Read the model definition and answer for the solid it produces. Units are mm, in the model's axes. A direction names the side the tool comes from. Coordinates: 2 decimals unless noted, no trailing zeros. Order: outer loops, then holes, each group sorted by start corner. A loop starts at its lowest first (then second) coordinate and runs counter-clockwise, first axis right, second up. Notation, with made-up numbers: (-23.5, 1.5) -> (5.5, 1.5) arc R29 ccw to (5.5, 31.5) -> close; hole circle Ø3 at (-18.75, 11). An arc over 180 degrees is marked (long way). Answer in a Markdown table with one row per item.
from build123d import *

# Parameters (mm, degrees)
SKETCH1_W           = 50
SKETCH1_H           = 25
BOSS_EXTRUDE1_DEPTH = 3
BOSS_EXTRUDE2_DEPTH = 42
SKETCH3_R           = 1.7
CUT_EXTRUDE1_DEPTH  = 71.774289117
FILLET2_R           = 4
FILLET3_R           = 4


with BuildPart() as part:
    # Sketch1 → Boss-Extrude1 (new body)
    with BuildSketch(Plane.XY):
        with Locations((25, -12.5)):
            Rectangle(SKETCH1_W, SKETCH1_H)
    extrude(amount=-BOSS_EXTRUDE1_DEPTH)

    # Sketch2 → Boss-Extrude2 (add)
    with BuildSketch(Plane(origin=(0, 0, -3), x_dir=(-1, 0, 0), z_dir=(0, 0, -1))):
        Polygon((-25, -25), (-29, -25), (-29, -22), (-25, -22), (-21, -22), (-21, -25), align=None)
    extrude(amount=BOSS_EXTRUDE2_DEPTH)

    # Sketch3 → Cut-Extrude1 (cut, through all)
    with BuildSketch(Plane(origin=(0, -22, 0), x_dir=(1, 0, 0), z_dir=(0, 1, 0))):
        with Locations(Location((25, 42, 0), (0, 0, 270))):
            Circle(SKETCH3_R)
        with Locations(Location((25, 15.3, 0), (0, 0, 270))):
            Circle(SKETCH3_R)
    extrude(amount=-CUT_EXTRUDE1_DEPTH, mode=Mode.SUBTRACT)

    # Fillet2
    fillet2_edges = [part.edges().sort_by_distance(p)[0] for p in [
        (29, -23.5, -45),
    ]]
    fillet(fillet2_edges, radius=FILLET2_R)

    # Fillet3
    fillet3_edges = [part.edges().sort_by_distance(p)[0] for p in [
        (21, -23.5, -45),
    ]]
    fillet(fillet3_edges, radius=FILLET3_R - 0.0001)  # a hair under: the kernel refuses the full size


solid = part.part
Q1. For faces 1 (the face through (25, -22, -24)), 2 (the face through (50, -13, -1)), 3 (the face through (21, -23, -22)), 4 (the face through (29, -24, -22)), determine the directions among +Z, -Z, +X, -X, +Y, -Y from which every point of the face is accessible in a straight line to the end or side of a thin tool.
Outcome:
| item | result |
|---|---|
| face 1 | -Z, +X, -X, +Y |
| face 2 | +Z, -Z, +X, +Y, -Y |
| face 3 | -Z, -X, +Y, -Y |
| face 4 | -Z, +X, +Y, -Y |
Q2. The part is cut by section C-C (y = -14.5). Write down the section's boundary in (x, z), then the cut area to 3 significant figures.
Outcome:
| item | result |
|---|---|
| outline | (0, -3) -> (50, -3) -> (50, 0) -> (0, 0) -> close |
| area | 150 mm² |
Q3. Given pin 1 (4.5 mm diameter, centred on x = 25, z = -42, fed in from +Y); pin 2 (1.5 mm diameter, centred on y = -23, z = -14, fed in from +X); pin 3 (7.5 mm diameter, centred on x = 26.5, y = -7, fed in from -Z), each flat-ended and moving along its own axis, determine where each tip first touches the part or whether it passes through.
Outcome:
| item | result |
|---|---|
| pin 1 | y = -22 |
| pin 2 | x = 29 |
| pin 3 | z = -3 |
Q4. The part is cut by section A-A (z = -15.3). Write down the section's boundary in (x, y), then the cut area to 3 significant figures.
Outcome:
| item | result |
|---|---|
| outline | (21, -25) -> (23.3, -25) -> (23.3, -22) -> (21, -22) -> close; (26.7, -25) -> (29, -25) -> (29, -22) -> (26.7, -22) -> close |
| area | 13.8 mm² |
Q5. The part is cut by section D-D (z = -42). Write down the section's boundary in (x, y), then the cut area to 3 significant figures.
Outcome:
| item | result |
|---|---|
| outline | (21.13, -25) -> (23.3, -25) -> (23.3, -22) -> (21.13, -22) -> close; (26.7, -25) -> (28.87, -25) -> (28.87, -22) -> (26.7, -22) -> close |
| area | 13.0 mm² |
Q6. For a pull along X with two mould halves and no side action, classify faces 5 (the face through (27.797, -23.479, -43.859)), 6 (the face through (25, -12, -3)), 7 (the face through (26.15, -23.48, -43.25)) as pulls with the +X half, pulls with the -X half, needs draft (parallel to the pull), parting line crosses it, or undercut.
Outcome:
| item | result |
|---|---|
| face 5 | pulls with the +X half |
| face 6 | needs draft |
| face 7 | undercut |
Q7. Consider line 1 (X direction, y = -23, z = -15.3); line 2 (Z direction, x = 38.5, y = -9.25); line 3 (X direction, y = -23.5, z = -35). Determine where each line is inside the solid, lowest interval first.
Outcome:
| item | result |
|---|---|
| line 1 | 21 to 23.3, 26.7 to 29 |
| line 2 | -3 to 0 |
| line 3 | 21 to 29 |
Q8. The part is cut by section B-B (x = 32). Write down the section's boundary in (y, z).
Outcome:
| item | result |
|---|---|
| outline | (-25, -3) -> (0, -3) -> (0, 0) -> (-25, 0) -> close |
